Input: dimensioned drawing with shaded views. Units: mm. Origin: part minimum x, y, z. Coordinates: 2 decimals unless noted, no trailing zeros. Order: outer loops, then holes, each group sorted by start corner. A loop starts at its lowest first (then second) coordinate and runs counter-clockwise, first axis right, second up. Notation, with made-up numbers: (-19, 51) - (2, 51) arc R14 cw to (2, 66) - close; hole circle Ø8 at (22.5, 39). An arc over 180 degrees is marked (long way). Answer as CSV lines item,"result". Start each with the question number.
Item 1: Material intervals for line 1 along Y through (x, z) = (59, 1.05); line 2 along Y through (x, z) = (15.5, 1.5); line 3 along Y through (x, z) = (25, 1.5), sorted ascending.
Item 2: Section C-C (y = 55). Output: boundary loops of the cut face in (x, z).
Item 3: Section A-A (y = 35.5). Output: boundary loops of the cut face in (x, z).
Item 4: First-contact query: pin 1 (2.5 mm diameter, centred on x = 5, y = 14.5, fed in from -Z); pin 2 (0.9 mm diameter, centred on y = 53.5, z = 1.5, fed in from -X). Flat tips, straight axial feed; report the tip coordinate or a pass-through.
Item 5: Section B-B (x = 15.5). Output: boundary loops of the cut face in (y, z), and give its area (3 significant figures).
Item 6: Section D-D (z = 1.9). State how many separate pieces and enclosed holes the cut face has, and give its area (3 significant figures).
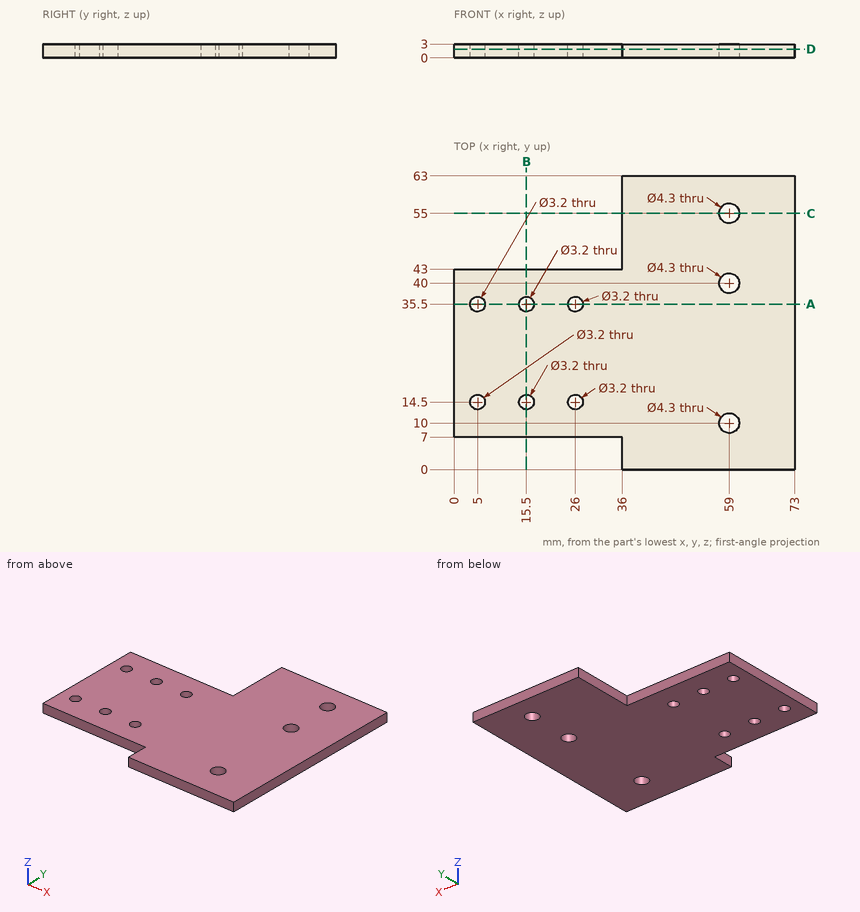
Determined:
1,line 1,"y = 0 to 7.85, 12.15 to 37.85, 42.15 to 52.85, 57.15 to 63"
1,line 2,"y = 7 to 12.9, 16.1 to 33.9, 37.1 to 43"
1,line 3,"y = 7 to 13.25, 15.75 to 34.25, 36.75 to 43"
2,outline,"(36, 0) - (56.85, 0) - (56.85, 3) - (36, 3) - close; (61.15, 0) - (73, 0) - (73, 3) - (61.15, 3) - close"
3,outline,"(0, 0) - (3.4, 0) - (3.4, 3) - (0, 3) - close; (6.6, 0) - (13.9, 0) - (13.9, 3) - (6.6, 3) - close; (17.1, 0) - (24.4, 0) - (24.4, 3) - (17.1, 3) - close; (27.6, 0) - (73, 0) - (73, 3) - (27.6, 3) - close"
4,pin 1,"passes through"
4,pin 2,"stops at x = 36"
5,outline,"(7, 0) - (12.9, 0) - (12.9, 3) - (7, 3) - close; (16.1, 0) - (33.9, 0) - (33.9, 3) - (16.1, 3) - close; (37.1, 0) - (43, 0) - (43, 3) - (37.1, 3) - close"
5,area,"88.8 mm^2"
6,separate pieces,"1"
6,enclosed holes,"9"
6,area,"3,540 mm^2"
